Part model, mm, in its own coordinate system. Coordinates: 2 decimals unless noted, no trailing zeros. Write each loop counter-clockwise with the first axis right and the second up, starting at its lowest first coordinate (ties: lowest second). Pieces come first, ordered by that corner, then holes. Notation, with made-up numbers: (17, 56.25) - (22, 56.25) arc R23 ccw to (22, 66.25) - close; hole circle Ø3 at (48, 13.5). An arc over 180 degrees is marked (long way). Write each question's results on one line, items separated by ' | '.
from build123d import *

# Parameters (mm, degrees)
BOSS_EXTRUDE1_DEPTH = 6.35
SKETCH2_W           = 88.9
SKETCH2_H           = 6.35
BOSS_EXTRUDE2_DEPTH = 6.35
FILLET1_R           = 2.54
BOSS_EXTRUDE3_DEPTH = 6.35


with BuildPart() as part:
    # Sketch1 → Boss-Extrude1 (new body)
    with BuildSketch(Plane(origin=(0, 0, 0), x_dir=(1, 0, 0), z_dir=(0, 1, 0))):
        with BuildLine():
            ThreePointArc((12.7, 0), (0, -12.7), (-12.7, 0))
            Line((-12.7, 0), (-12.7, -127))
            Line((-12.7, -127), (12.7, -127))
            Line((12.7, -127), (12.7, 0))
        make_face()
        with BuildLine():
            ThreePointArc((12.7, 0), (0, 12.7), (-12.7, 0))
            Line((-12.7, 0), (12.7, 0))
        make_face()
        with BuildLine():
            Line((12.7, 0), (-12.7, 0))
            ThreePointArc((-12.7, 0), (0, -12.7), (12.7, 0))
        make_face()
    extrude(amount=BOSS_EXTRUDE1_DEPTH)

    # Sketch2 → Boss-Extrude2 (add)
    with BuildSketch(Plane(origin=(0, 6.35, 0), x_dir=(1, 0, 0), z_dir=(0, 1, 0))):
        with Locations((31.75, -130.175)):
            Rectangle(SKETCH2_W, SKETCH2_H)
    extrude(amount=-BOSS_EXTRUDE2_DEPTH)

    # Fillet1
    fillet1_edges = [part.edges().sort_by_distance(p)[0] for p in [
        (12.7, 3.175, 127),
    ]]
    fillet(fillet1_edges, radius=FILLET1_R)

    # Sketch3 → Boss-Extrude3 (add)
    with BuildSketch(Plane(origin=(0, 0, 0), x_dir=(-1, 0, 0), z_dir=(0, -1, 0))):
        with BuildLine():
            Line((-7.384124229, 1.213847931), (7.384124229, 1.213847931))
            Line((7.384124229, 1.213847931), (5.698055631, 17.468424552))
            ThreePointArc((5.698055631, 17.468424552), (0, 22.606), (-5.698055631, 17.468424552))
            Line((-5.698055631, 17.468424552), (-7.384124229, 1.213847931))
        make_face()
    extrude(amount=-BOSS_EXTRUDE3_DEPTH)


solid = part.part
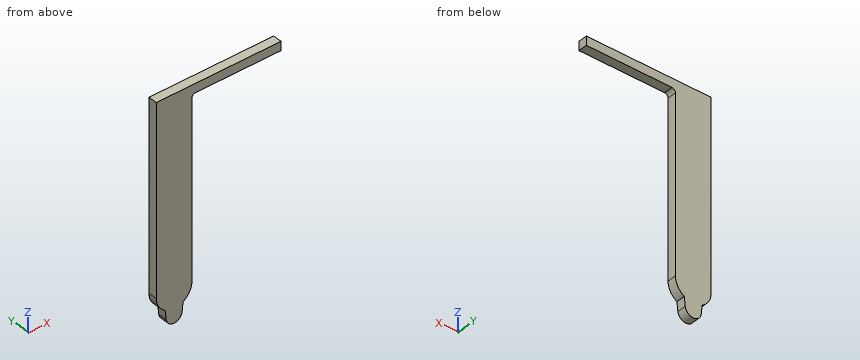
(1) Saw through at B-B on z = 65.5. Write the cut outline in (x, y), then the cut area to 3 significant figures.
Return value:
outline: (-12.7, 0) - (12.7, 0) - (12.7, 6.35) - (-12.7, 6.35) - close | area: 161 mm^2
(2) Saw through at A-A on y = 3.25. Write the cut outline in (x, z), then the cut area to 3 significant figures.
Return value:
outline: (-12.7, 0) arc R12.7 ccw to (-6.37, -10.99) - (-5.7, -17.47) arc R5.73 ccw to (5.7, -17.47) - (6.37, -10.99) arc R12.7 ccw to (12.7, 0) - (12.7, 124.46) arc R2.54 cw to (15.24, 127) - (76.2, 127) - (76.2, 133.35) - (-12.7, 133.35) - close | area: 4,150 mm^2
(3) Wall check: line 1 (X direction, y = 1.75, z = 95); line 2 (Z direction, x = 18, y = 2.75); line 3 (Z direction, x = -7.5, y = 2.75). Give the ranges that are in metal, low to high. Write a range as from..to.
Return value:
line 1: x = -12.7..12.7 | line 2: z = 127..133.35 | line 3: z = -10.25..133.35
(4) Flat gauge pin, fed straight in: P1, Ø2, axis at x = 46, y = 3.5, coming from the -Z side. Where does the tip first touch, or does it go through?
Return value:
P1: stops at z = 127
(5) Saw through at C-C on x = 28. Write the cut outline in (y, z).
Return value:
outline: (0, 127) - (6.35, 127) - (6.35, 133.35) - (0, 133.35) - close
